Design review of the part built by this model. Coordinates are the model's own, in mm. Face numbers are marked on the shaded views. Coordinates: 2 decimals unless noted, no trailing zeros. Loops run counter-clockwise (first coordinate to the right, second up) from the corner with the lowest first, then second, coordinate; pieces in that order, holes last. Notation, with made-up numbers: (60, 14) -> (72, 14) arc R11 cw to (72, 29) -> close; hole circle Ø9 at (17, 72). An arc over 180 degrees is marked (long way). Use a Markdown table: item, result. Add a question column.
Q1. Take a section at B-B on x = -21. Write out the cut boundary in (y, z).
Q2. Take a section at A-A on z = 15. Count the separate pieces of the cut face and the enclosed holes in it, plus the area to 3 significant figures.
Q3. For probe 1 along Y at (x, z) = (0, 2.1); probe 2 along Y at (x, z) = (12.5, 28); probe 3 along Y at (x, z) = (1, 14.75), list the stretches that pass through material, from the lowest coordinate up.
Q4. Take a section at D-D on x = 14. Write out the cut boundary in (y, z), plus the area to 3 significant figures.
Q5. Take a section at C-C on y = -26. Write out the cut boundary in (x, z), plus the area to 3 significant figures.
Q6. Clearance check with flat-ended pins moving along their axes: pin 1 Ø4 at (y, z) = (3.5, 12) entering from -X; pin 2 Ø6 at (y, z) = (8, 22.5) entering from -X; pin 3 Ø1 at (x, z) = (-4, 4) entering from +Y. State where each tip first meets the part, or that it passes through.
Q7. Draft analysis for pull direction Y (two halves, no side actions). For the marked faces 1, 2 and 3, state which applies: pulls with the +Y half, pulls with the -Y half, needs draft (parallel to the pull), parting line crosses it, or undercut.
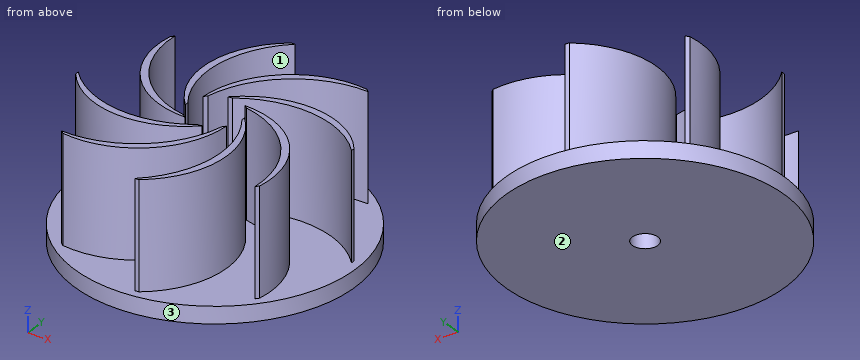
from build123d import *

# Parameters (mm, degrees)
SKETCH1_R           = 33.274
BOSS_EXTRUDE1_DEPTH = 4
SKETCH2_R           = 3.048
CUT_EXTRUDE1_DEPTH  = 5
BOSS_EXTRUDE2_DEPTH = 25.4
SKETCH4_R           = 6.35
CUT_EXTRUDE2_DEPTH  = 56.896
SKETCH5_R           = 33.274
SKETCH5_R_2         = 31.253208268
CUT_EXTRUDE3_DEPTH  = 120.142


with BuildPart() as part:
    # Sketch1 → Boss-Extrude1 (new body)
    with BuildSketch(Plane.XY):
        Circle(SKETCH1_R)
    extrude(amount=BOSS_EXTRUDE1_DEPTH)

    # Sketch2 → Cut-Extrude1 (cut, through all)
    with BuildSketch(Plane.XY.offset(4)):
        Circle(SKETCH2_R)
    extrude(amount=-CUT_EXTRUDE1_DEPTH, mode=Mode.SUBTRACT)

    # Sketch3 → Boss-Extrude2 (add)
    with BuildSketch(Plane.XY.offset(4)):
        with BuildLine():
            ThreePointArc((5.08, 0), (-2.558445785, -19.86901744), (-23.528271037, -23.528271037))
            ThreePointArc((-23.528271037, -23.528271037), (-3.66763311, -18.52034496), (5.08, 0))
        make_face()
        with BuildLine():
            ThreePointArc((3.592102448, -3.592102448), (-15.689269754, -10.502453268), (-33.274, 0))
            ThreePointArc((-33.274, 0), (-15.858611331, -12.240422604), (3.592102448, -3.592102448))
        make_face()
        with BuildLine():
            ThreePointArc((0, -5.08), (-19.86901744, 2.558445785), (-23.528271037, 23.528271037))
            ThreePointArc((-23.528271037, 23.528271037), (-18.52034496, 3.66763311), (0, -5.08))
        make_face()
        with BuildLine():
            ThreePointArc((-3.592102448, -3.592102448), (-12.240422604, 15.858611331), (0, 33.274))
            ThreePointArc((0, 33.274), (-10.502453268, 15.689269754), (-3.592102448, -3.592102448))
        make_face()
        with BuildLine():
            ThreePointArc((-5.08, 0), (2.558445785, 19.86901744), (23.528271037, 23.528271037))
            ThreePointArc((23.528271037, 23.528271037), (3.66763311, 18.52034496), (-5.08, 0))
        make_face()
        with BuildLine():
            ThreePointArc((-3.592102448, 3.592102448), (15.858611331, 12.240422604), (33.274, 0))
            ThreePointArc((33.274, 0), (15.689269754, 10.502453268), (-3.592102448, 3.592102448))
        make_face()
        with BuildLine():
            ThreePointArc((0, 5.08), (19.86901744, -2.558445785), (23.528271037, -23.528271037))
            ThreePointArc((23.528271037, -23.528271037), (18.52034496, -3.66763311), (0, 5.08))
        make_face()
        with BuildLine():
            ThreePointArc((3.592102448, 3.592102448), (12.240422604, -15.858611331), (0, -33.274))
            ThreePointArc((0, -33.274), (10.502453268, -15.689269754), (3.592102448, 3.592102448))
        make_face()
    extrude(amount=BOSS_EXTRUDE2_DEPTH)

    # Sketch4 → Cut-Extrude2 (cut)
    with BuildSketch(Plane.XY.offset(4)):
        Circle(SKETCH4_R)
    extrude(amount=CUT_EXTRUDE2_DEPTH, mode=Mode.SUBTRACT)

    # Sketch5 → Cut-Extrude3 (cut)
    with BuildSketch(Plane.XY.offset(4)):
        Circle(SKETCH5_R)
        Circle(SKETCH5_R_2, mode=Mode.SUBTRACT)
    extrude(amount=CUT_EXTRUDE3_DEPTH, mode=Mode.SUBTRACT)


solid = part.part
Answer list:
| question | item | result |
|---|---|---|
| 1 | outline | (-25.81, 0) -> (25.81, 0) -> (25.81, 4) -> (7.32, 4) -> (7.32, 29.4) -> (4.06, 29.4) -> (4.06, 4) -> (-9.37, 4) -> (-9.37, 29.4) -> (-11.09, 29.4) -> (-11.09, 4) -> (-25.81, 4) -> close |
| 2 | separate pieces | 8 |
| 2 | enclosed holes | 0 |
| 2 | area | 381 mm² |
| 3 | probe 1 | -33.27 to -3.05, 3.05 to 33.27 |
| 3 | probe 2 | 1.56 to 3.21, 10.6 to 12.31, 23.11 to 24.45 |
| 3 | probe 3 | -16.15 to -13.38, -6.5 to -6.27, 7.18 to 8.16, 15.96 to 18.45 |
| 4 | outline | (-30.19, 0) -> (30.19, 0) -> (30.19, 4) -> (24.66, 4) -> (24.66, 29.4) -> (23.47, 29.4) -> (23.47, 4) -> (12.34, 4) -> (12.34, 29.4) -> (10.61, 29.4) -> (10.61, 4) -> (2.42, 4) -> (2.42, 29.4) -> (0.57, 29.4) -> (0.57, 4) -> (-30.19, 4) -> close |
| 4 | area | 363 mm² |
| 5 | outline | (-20.76, 0) -> (20.76, 0) -> (20.76, 4) -> (8.54, 4) -> (8.54, 29.4) -> (7.02, 29.4) -> (7.02, 4) -> (-20.76, 4) -> close |
| 5 | area | 205 mm² |
| 6 | pin 1 | x = -21.9 |
| 6 | pin 2 | x = -24.13 |
| 6 | pin 3 | y = 33.09 |
| 7 | face 1 | undercut |
| 7 | face 2 | needs draft |
| 7 | face 3 | parting line crosses it |
